Autodesk Inventor part; units mm, degrees
ref_plane "Work Plane1" through (0, 0, 100) normal (0, 0, -1) x (-1, 0, 0)
ref_plane "axialPlane" through (0, -10.5, 0) normal (1, 0, 0) x (0, 0, -1)
ref_plane "YZ Plane" through (0, 0, 0) normal (1, 0, 0) x (0, 1, 0)
sketch "Sketch1" plane through (0, 0, 0) normal (0, 0, 1) x (1, 0, 0)
  line L0 (-12.5, 12.5) -> (12.5, 12.5)
  line L1 (12.5, 12.5) -> (12.5, -12.5)
  line L2 (12.5, -12.5) -> (-12.5, -12.5)
  line L3 (-12.5, -12.5) -> (-12.5, 12.5)
  line L4 (10, 10) -> (-10, 10)
  line L5 (-10, 10) -> (-10, -10)
  line L6 (-10, -10) -> (10, -10)
  line L7 (10, -10) -> (10, 10)
  point P0 (0, 0)
  dimension "d0" = 25
  dimension "d1" = 25
  dimension "d2" = 12.5
  dimension "d3" = 12.5
  dimension "d4" = 2.5
extrude "Extrusion1" add sketch "Sketch1" along normal blind 1000
fillet "Fillet1" radius 2 4 edges at (12.5, 12.5, 500) (-12.5, 12.5, 500) (-12.5, -12.5, 500) (12.5, -12.5, 500)
ref_plane "Work Plane1" through (0, 0, 100) normal (0, 0, -1) x (-1, 0, 0)
split "Split1" plane through (0, 0, 100) removes the side toward (0, 0, 1)
ref_plane "axialPlane" through (0, -10.5, 0) normal (1, 0, 0) x (0, 0, -1)
equation "\"d0\" = -2 * a + sm_varx_squareBarDimension - tol"
equation "\"d1\" = d0"
equation "\"d4\" = sm_varx_squareBarThickness"
equation "\"sm_varx_squareBarThickness\" = 2.5"
equation "\"a\" = sm_varx_squareBarThickness"
equation "\"hoop_angle_z\" = 45deg"
equation "\"hoop_bearing_length\" = 5deg"
equation "\"hoop_cable_diam\" = 5"
equation "\"hoop_cable_pulley_diam\" = 22"
equation "\"hoop_thickness_large\" = 4"
equation "\"hoop_thickness_medium\" = 3.2"
equation "\"hoop_thickness_small\" = 2"
equation "\"hoop_width_large\" = 51"
equation "\"hoop_width_medium\" = 33.7"
equation "\"hoop_width_small\" = 25.4"
equation "\"rack_tooth_addendum\" = 5"
equation "\"rack_tooth_dedendum\" = 5"
equation "\"rack_tooth_thickness\" = 5"
equation "\"secure_arm_angle\" = 35deg"
equation "\"secure_arm_radii\" = 9"
equation "\"support_baseClamp_platformLengthBuffer\" = 35"
equation "\"support_baseClamp_platformThickness\" = 15"
equation "\"support_baseClamp_platformWidthBuffer\" = 0"
equation "\"support_baseClamp_sleeveHoleDiameter\" = 12"
equation "\"support_baseClamp_sleeveSweepTerminationAngle\" = 55deg"
equation "\"support_baseClamp_thickness\" = 8"
equation "\"support_frame_endHoleBuffer\" = 45"
equation "\"support_frame_squareBarFillet\" = 2"
equation "\"support_frame_squareBarThickness\" = 5"
equation "\"hoop_tabs_thickness\" = 6"
equation "\"hoop_tabs_hole\" = 12"
equation "\"wheelchair_deployed_width\" = 635"
equation "\"wheelchair_deployed_length\" = 1067"
equation "\"wheelchair_deployed_height\" = 914"
equation "\"sm_varx_pinPlate_thickness\" = 5"
equation "\"sm_varx_pinPlate_holeDiameter\" = 5"
equation "\"sm_varx_member_tolerance\" = 0"
equation "\"hoop_bushing12_radialInterference\" = 0"
equation "\"hoop_bushing23_radialInterference\" = 0"
equation "\"hoop_bushing23_od\" = -2 * hoop_thickness_medium + hoop_width_medium + hoop_bushing23_radialInterference"
equation "\"hoop_bushing23_thickness\" = -hoop_width_small + hoop_bushing23_od - 2 * hoop_bushing23_radialInterference"
equation "\"hoop_bushing12_od\" = -2 * hoop_thickness_large + hoop_width_large + hoop_bushing12_radialInterference"
equation "\"wheelchatir_pos_deploy_angle_0\" = 65deg"
equation "\"wheelchatir_pos_store_angle_0\" = 90deg"
equation "\"wheelchatir_pos_deploy_angle_1\" = 20deg"
equation "\"wheelchatir_pos_store_angle_1\" = 20deg"
equation "\"hoop_bushing12_thickness\" = -hoop_width_medium + hoop_bushing12_od - 2 * hoop_bushing12_radialInterference"
properties part number "member_axial" material "Steel, Galvanized"
Verification items for the finished model (mm, model axes). A direction names the side the tool comes from. Give positions to 0.01 mm unless a question says otherwise; leave off trailing zeros. Loops run counter-clockwise (first coordinate to the right, second up) from the corner with the lowest first, then second, coordinate; pieces in that order, holes last.
1. Mould release check, pull along X, two halves, no side actions. Record for faces 1 (the flat face through (-12.5, 0, 49)), 2 (the flat face through (-10, 0, 49)), 3 (the cylindrical face through (11.9, -11.93, 50.7)), 4 (the flat face through (0, -12.5, 49)): released by +X, released by -X, zero draft, split by the parting line, or undercut.
2. Thickness scan on line 1 (X direction, y = -0.25, z = 51); line 2 (X direction, y = 10.75, z = 36.5). Record the ranges inside material, lowest first.
3. Section check B-B, the plane z = 78. Enter the section's corners in (x, y).
4. Set-up check for faces 5 (the flat face through (0, 12.5, 49)), 6 (the flat face through (0, -10, 49)): record each of +Z, -Z, +X, -X, +Y, -Y from which the full face is reachable in a straight line by a thin tool's end or side.
5. Go/stop test with a flat-tipped pin: pin 1 Ø5 at (x, y) = (-6, 9) entering from +Z. Record where the tip stops, or that it passes through.
6. Section check A-A, the plane y = -7.5. Enter the section's corners in (x, z), then the cut area to 3 significant figures.
Geometry says:
1. face 1: released by -X
1. face 2: undercut
1. face 3: released by +X
1. face 4: zero draft
2. line 1: x = -12.5 to -10, 10 to 12.5
2. line 2: x = -12.48 to 12.48
3. outline: (-12.5, -10.5) arc R2 ccw to (-10.5, -12.5) - (10.5, -12.5) arc R2 ccw to (12.5, -10.5) - (12.5, 10.5) arc R2 ccw to (10.5, 12.5) - (-10.5, 12.5) arc R2 ccw to (-12.5, 10.5) - close; hole (-10, -10) - (10, -10) - (10, 10) - (-10, 10) - close
4. face 5: +Z, -Z, +X, -X, +Y
4. face 6: +Z, -Z
5. pin 1: stops at z = 100
6. outline: (-12.5, 0) - (-10, 0) - (-10, 100) - (-12.5, 100) - close; (10, 0) - (12.5, 0) - (12.5, 100) - (10, 100) - close
6. area: 500 mm2
